Geometry: final body of the model. Coordinates: model frame, mm. Face numbers are marked on the shaded views. A direction names the side the tool comes from. Give positions to 0.01 mm unless a question says otherwise; leave off trailing zeros. Write each loop counter-clockwise with the first axis right and the second up, starting at its lowest first coordinate (ties: lowest second). Pieces come first, ordered by that corner, then holes. Notation, with made-up numbers: (48, 5) - (82, 5) arc R22 ccw to (82, 35) - close; hole circle Ø6 at (-16.5, -17.5). An arc over 180 degrees is marked (long way). One line per question, with ' | ' between items. Start each with the question number.
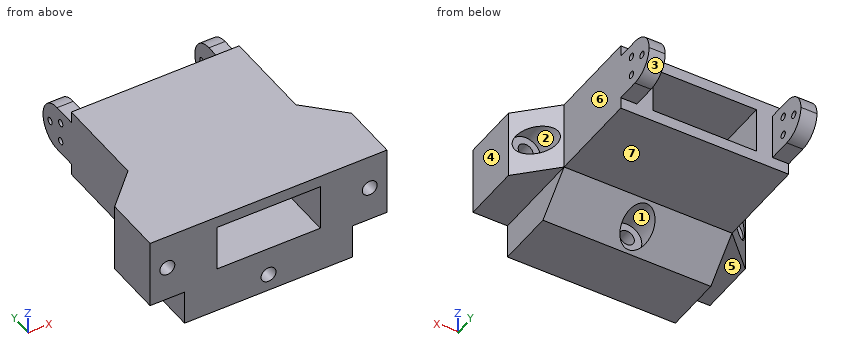
```python
from build123d import *

# Parameters (mm, degrees)
BOSS_EXTRUDE1_DEPTH = 30
SKETCH2_R           = 3.25
SKETCH2_W           = 45
SKETCH2_H           = 20
CUT_EXTRUDE1_DEPTH  = 90
SKETCH3_W           = 7
SKETCH3_H           = 20
BOSS_EXTRUDE2_DEPTH = 20
SKETCH4_R           = 1.5
CUT_EXTRUDE2_DEPTH  = 80
FILLET1_R           = 10
CUT_EXTRUDE3_START  = -25
SKETCH5_R           = 6.5
CUT_EXTRUDE3_DEPTH  = 17
BOSS_EXTRUDE3_DEPTH = 73
SKETCH7_R           = 3.25
CUT_EXTRUDE4_DEPTH  = 40
CUT_EXTRUDE5_START  = -25
SKETCH8_R           = 6.5
CUT_EXTRUDE5_DEPTH  = 17


with BuildPart() as part:
    # Sketch1 → Boss-Extrude1 (new body)
    with BuildSketch(Plane.XY):
        Polygon((0, 40), (-15, 25), (-15, 0), (0, 0), (73, 0), (88, 0), (88, 25), (73, 40), (73, 80), (0, 80), align=None)
    extrude(amount=BOSS_EXTRUDE1_DEPTH)

    # Sketch2 → Cut-Extrude1 (cut)
    with BuildSketch(Plane.XZ):
        with Locations(Location((-7.5, 15, 0), (0, 0, 270))):
            Circle(SKETCH2_R)
        with Locations(Location((80.5, 15, 0), (0, 0, 270))):
            Circle(SKETCH2_R)
        with Locations((36.5, 15)):
            Rectangle(SKETCH2_W, SKETCH2_H)
    extrude(amount=-CUT_EXTRUDE1_DEPTH, mode=Mode.SUBTRACT)

    # Sketch3 → Boss-Extrude2 (add)
    with BuildSketch(Plane(origin=(0, 80, 0), x_dir=(1, 0, 0), z_dir=(0, 1, 0))):
        with Locations((3.5, -15)):
            Rectangle(SKETCH3_W, SKETCH3_H)
        with Locations((69.5, -15)):
            Rectangle(SKETCH3_W, SKETCH3_H)
    extrude(amount=BOSS_EXTRUDE2_DEPTH)

    # Sketch4 → Cut-Extrude2 (cut)
    with BuildSketch(Plane(origin=(73, 0, 0), x_dir=(0, 0, -1), z_dir=(1, 0, 0))):
        with Locations((-15, 95)):
            Circle(SKETCH4_R)
        with Locations((-10.669872981, 87.5)):
            Circle(SKETCH4_R)
        with Locations((-19.330127019, 87.5)):
            Circle(SKETCH4_R)
    extrude(amount=-CUT_EXTRUDE2_DEPTH, mode=Mode.SUBTRACT)

    # Fillet1
    fillet1_edges = [part.edges().sort_by_distance(p)[0] for p in [
        (3.5, 100, 25),
        (69.5, 100, 25),
        (3.5, 100, 5),
        (69.5, 100, 5),
    ]]
    fillet(fillet1_edges, radius=FILLET1_R - 0.0001)  # a hair under: the kernel refuses the full size

    # Sketch5 → Cut-Extrude3 (cut)
    with BuildSketch(Plane.XZ.offset(CUT_EXTRUDE3_START)):
        with Locations(Location((-7.5, 15, 0), (0, 0, 270))):
            Circle(SKETCH5_R)
        with Locations(Location((80.5, 15, 0), (0, 0, 270))):
            Circle(SKETCH5_R)
    extrude(amount=-CUT_EXTRUDE3_DEPTH, mode=Mode.SUBTRACT)

    # Sketch6 → Boss-Extrude3 (add)
    with BuildSketch(Plane(origin=(0, 0, 0), x_dir=(0, 0, -1), z_dir=(1, 0, 0))):
        Polygon((0, 40), (0, 0), (15, 0), (15, 25), align=None)
    extrude(amount=BOSS_EXTRUDE3_DEPTH)

    # Sketch7 → Cut-Extrude4 (cut)
    with BuildSketch(Plane.XZ):
        with Locations(Location((36.5, -7.5, 0), (0, 0, 270))):
            Circle(SKETCH7_R)
    extrude(amount=-CUT_EXTRUDE4_DEPTH, mode=Mode.SUBTRACT)

    # Sketch8 → Cut-Extrude5 (cut)
    with BuildSketch(Plane.XZ.offset(CUT_EXTRUDE5_START)):
        with Locations(Location((36.5, -7.5, 0), (0, 0, 270))):
            Circle(SKETCH8_R)
    extrude(amount=-CUT_EXTRUDE5_DEPTH, mode=Mode.SUBTRACT)


solid = part.part
```
1) First-contact query: pin 1 Ø6 at (x, z) = (66.5, 7.5) entering from +Y; pin 2 Ø2 at (x, y) = (70, 85.5) entering from -Z; pin 3 Ø14.5 at (x, z) = (37.5, -4.5) entering from +Y; pin 4 Ø5 at (x, z) = (80.5, 15) entering from -Y. Flat tips, straight axial feed; report the tip coordinate or a pass-through.
2) Section D-D, the plane z = -7.5. Output: boundary loops of the cut face in (x, y).
3) Line query: L1, parallel to X at y = 10, z = 15; L2, parallel to Z at x = 71.25, y = 87.5; L3, parallel to Z at x = 52, y = 67. Output: solid intervals per line, ascending.
4) Section B-B, the plane y = 87.5. Output: boundary loops of the cut face in (x, z), plus the area to 3 significant figures.
5) Pull-direction query (Z, two-part tool) for the marked faces 1, 2, 3 and 4; classes: +Z half, -Z half, draft (parallel to the pull), parting line (faces both ways), or undercut.
6) Section A-A, the plane x = 36.5. Output: boundary loops of the cut face in (y, z), plus the area to 3 significant figures.
7) Section C-C, the plane x = -7.5. Output: boundary loops of the cut face in (y, z).
8) Reachability of the marked faces 5, 6 and 7 from +Z, -Z, +X, -X, +Y, -Y: full face, straight path, thin tool, end or side. Return the list, or none.
Answer key:
1) pin 1: y = 98.93 | pin 2: z = 5 | pin 3: y = 80 | pin 4: through
2) outline: (0, 0) - (33.25, 0) - (33.25, 25) - (30, 25) - (30, 32.5) - (0, 32.5) - close; (39.75, 0) - (73, 0) - (73, 32.5) - (43, 32.5) - (43, 25) - (39.75, 25) - close
3) L1: -15 to -10.75, -4.25 to 14, 59 to 77.25, 83.75 to 88 | L2: 5 to 9.17, 12.17 to 17.83, 20.83 to 25 | L3: 0 to 5, 25 to 30
4) outline: (0, 5) - (7, 5) - (7, 9.17) - (0, 9.17) - close; (0, 12.17) - (7, 12.17) - (7, 17.83) - (0, 17.83) - close; (0, 20.83) - (7, 20.83) - (7, 25) - (0, 25) - close; (66, 5) - (73, 5) - (73, 9.17) - (66, 9.17) - close; (66, 12.17) - (73, 12.17) - (73, 17.83) - (66, 17.83) - close; (66, 20.83) - (73, 20.83) - (73, 25) - (66, 25) - close | area: 196 mm^2
5) face 1: undercut | face 2: undercut | face 3: -Z half | face 4: draft
6) outline: (0, -15) - (25, -15) - (26, -14) - (25, -14) - (25, -10.75) - (0, -10.75) - close; (0, -4.25) - (25, -4.25) - (25, -1) - (39, -1) - (40, 0) - (80, 0) - (80, 5) - (0, 5) - close; (0, 25) - (80, 25) - (80, 30) - (0, 30) - close | area: 1,030 mm^2
7) outline: (0, 0) - (32.5, 0) - (32.5, 8.5) - (25, 8.5) - (25, 11.75) - (0, 11.75) - close; (0, 18.25) - (25, 18.25) - (25, 21.5) - (32.5, 21.5) - (32.5, 30) - (0, 30) - close
8) face 5: -Z, -X, +Y, -Y | face 6: +Z, -Z, +X, +Y | face 7: -Z, +X, -X, +Y
